The model under review builds one solid part; all positions refer to its coordinate system, in mm. A direction names the side the tool comes from. Coordinates: 2 decimals unless noted, no trailing zeros. Order: outer loops, then holes, each group sorted by start corner. A loop starts at its lowest first (then second) coordinate and runs counter-clockwise, first axis right, second up. Notation, with made-up numbers: M 63.25,19.5 L 118.25,19.5 A29 cw 118.25,42.5 Z; hole C 16,38.5 d3. An arc over 180 degrees is marked long. One line per item, written item: value.
```python
from build123d import *

# Parameters (mm, degrees)
EXTRUDE_1_DEPTH     = 30
SKETCH_2_R          = 10.25
CUT_EXTRUDE_1_DEPTH = 30
FILLET_2_R          = 1
FILLET_3_R          = 1
FILLET_4_R          = 1
FILLET_5_R          = 1


with BuildPart() as part:
    # Эскиз1 → Бобышка-Вытянуть1 (new body)
    with BuildSketch(Plane.XY):
        Polygon((-20, 7.029837238), (-20, 34.029837238), (0, 34.029837238), (0, -102.970162762), (3, -102.970162762), (3, 37.029837238), (-23, 37.029837238), (-23, 7.029837238), align=None)
    extrude(amount=EXTRUDE_1_DEPTH)

    # Эскиз2 → Вырез-Вытянуть1 (cut)
    with BuildSketch(Plane(origin=(3, 0, 0), x_dir=(0, 0, -1), z_dir=(1, 0, 0))):
        with Locations((-15, -82.970162762)):
            Circle(SKETCH_2_R)
    extrude(amount=-CUT_EXTRUDE_1_DEPTH, mode=Mode.SUBTRACT)

    # Скругление2
    fillet_2_edges = [part.edges().sort_by_distance(p)[0] for p in [
        (1.5, -102.970162762, 30),
    ]]
    fillet(fillet_2_edges, radius=FILLET_2_R)

    # Скругление3
    fillet_3_edges = [part.edges().sort_by_distance(p)[0] for p in [
        (1.5, -102.970162762, 0),
    ]]
    fillet(fillet_3_edges, radius=FILLET_3_R)

    # Скругление4
    fillet_4_edges = [part.edges().sort_by_distance(p)[0] for p in [
        (-21.5, 7.029837238, 30),
    ]]
    fillet(fillet_4_edges, radius=FILLET_4_R)

    # Скругление5
    fillet_5_edges = [part.edges().sort_by_distance(p)[0] for p in [
        (-21.5, 7.029837238, 0),
    ]]
    fillet(fillet_5_edges, radius=FILLET_5_R)


solid = part.part
```
(1) For L1, parallel to Y at x = 2.2, z = 15; L2, parallel to Y at x = -15, z = 13.5; L3, parallel to Y at x = -21.5, z = 4.25, list the stretches that pass through material, from the lowest coordinate up.
Geometry results:
L1: y = -102.97 to -93.22, -72.72 to 37.03
L2: y = 34.03 to 37.03
L3: y = 7.03 to 37.03
(2) We need section B-B, the plane z = 20.25. State the section outline as (x, y) points.
Geometry results:
outline: M -23,7.03 L -20,7.03 L -20,34.03 L 0,34.03 L 0,-74.17 L 3,-74.17 L 3,37.03 L -23,37.03 Z; M 0,-102.97 L 3,-102.97 L 3,-91.77 L 0,-91.77 Z
(3) Mouldability with a two-part tool opening along X and no side actions: class faces 4 (the flat face through (-23, 22, 15)), 5 (the flat face through (-20, 20, 15)), 6 (the flat face through (3, -34, 15)) as +X half, -X half, draft (parallel to the pull), parting line (faces both ways), or undercut.
Geometry results:
face 4: -X half
face 5: undercut
face 6: +X half
(4) We need section C-C, the plane y = -30. State the section outline as (x, z) points, plus the area to 3 significant figures.
Geometry results:
outline: M 0,0 L 3,0 L 3,30 L 0,30 Z
area: 90.0 mm2
(5) We need section D-D, the plane x = -2.25. State the section outline as (y, z) points.
Geometry results:
outline: M 34.03,0 L 37.03,0 L 37.03,30 L 34.03,30 Z
(6) Tool access review of faces 1 (the flat face through (-10, 34.03, 15)), 2 (the cylindrical face through (1.521, -74.327, 9.49)), 3 (the flat face through (-22, 7.03, 15)): name each direction out of +Z, -Z, +X, -X, +Y, -Y from which nothing blocks a thin tool from reaching the whole face with its end or side.
Geometry results:
face 1: +Z, -Z, -Y
face 2: +X, -X
face 3: +Z, -Z, -X, -Y
(7) We need section A-A, the plane z = 15. State the section outline as (x, y) points.
Geometry results:
outline: M -23,7.03 L -20,7.03 L -20,34.03 L 0,34.03 L 0,-72.72 L 3,-72.72 L 3,37.03 L -23,37.03 Z; M 0,-102.97 L 3,-102.97 L 3,-93.22 L 0,-93.22 Z
(8) Insertion check: pin 1 Ø1.5 at (x, z) = (-15, 10) entering from -Y; pin 2 Ø2.5 at (x, z) = (-21, 17.5) entering from -Y. Each pin has a flat end and moves straight along its axis. Give the tip position at first contact, or say it passes through.
Geometry results:
pin 1: stops at y = 34.03
pin 2: stops at y = 7.03
